```python
from build123d import *

# Parameters (mm, degrees)
SKETCH1_W           = 307
SKETCH1_H           = 115
BOSS_EXTRUDE1_DEPTH = 4
CUT_EXTRUDE1_DEPTH  = 4
SKETCH3_W           = 4
SKETCH3_H           = 40.5
SKETCH3_H_2         = 38.5
CUT_EXTRUDE2_DEPTH  = 4
SKETCH4_W           = 46.333333333
SKETCH4_H           = 4
SKETCH4_W_2         = 42.33
BOSS_EXTRUDE3_DEPTH = 4
SKETCH5_W           = 36
SKETCH5_H           = 4
BOSS_EXTRUDE4_DEPTH = 4
SKETCH7_W           = 22.24
SKETCH7_H           = 4
BOSS_EXTRUDE6_DEPTH = 4
SKETCH8_W           = 4
SKETCH8_H           = 38
CUT_EXTRUDE3_DEPTH  = 4
LPATTERN1_COUNT     = 3
LPATTERN1_PITCH     = 72
SKETCH9_W           = 70
SKETCH9_H           = 4
BOSS_EXTRUDE7_DEPTH = 4
CUT_EXTRUDE4_DEPTH  = 4
LPATTERN2_COUNT     = 2
LPATTERN2_PITCH     = 84
LPATTERN3_COUNT     = 2
LPATTERN3_PITCH     = 194
SKETCH11_W          = 4
SKETCH11_H          = 3.457617008
BOSS_EXTRUDE8_DEPTH = 4


with BuildPart() as part:
    # Sketch1 → Boss-Extrude1 (new body)
    with BuildSketch(Plane(origin=(0, 0, 0), x_dir=(0, 0, -1), z_dir=(1, 0, 0))):
        with Locations((153.5, 57.5)):
            Rectangle(SKETCH1_W, SKETCH1_H)
    extrude(amount=BOSS_EXTRUDE1_DEPTH)

    # Sketch2 → Cut-Extrude1 (cut)
    with BuildSketch(Plane.ZY):
        with BuildLine():
            Line((-78.216729868, 30.591924331), (-78.216729868, 118.288831206))
            Line((-78.216729868, 118.288831206), (-68.216729868, 118.288831206))
            Line((-68.216729868, 118.288831206), (-68.216729868, 30.591924331))
            ThreePointArc((-68.216729868, 30.591924331), (-73.216729868, 25.591924331), (-78.216729868, 30.591924331))
        make_face()
    extrude(amount=-CUT_EXTRUDE1_DEPTH, mode=Mode.SUBTRACT)

    # Sketch3 → Cut-Extrude2 (cut)
    with BuildSketch(Plane.ZY):
        with Locations((-2, 16.25)):
            Rectangle(SKETCH3_W, SKETCH3_H)
        with Locations((-2, 95.75)):
            Rectangle(SKETCH3_W, SKETCH3_H_2)
    extrude(amount=-CUT_EXTRUDE2_DEPTH, mode=Mode.SUBTRACT)

    # Sketch4 → Boss-Extrude3 (add)
    with BuildSketch(Plane.ZY):
        with Locations((-283.833333334, -2)):
            Rectangle(SKETCH4_W, SKETCH4_H)
        with Locations((-25.165, -2)):
            Rectangle(SKETCH4_W_2, SKETCH4_H)
    extrude(amount=-BOSS_EXTRUDE3_DEPTH)

    # Sketch5 → Boss-Extrude4 (add)
    with BuildSketch(Plane.ZY):
        with Locations((-271, 117)):
            Rectangle(SKETCH5_W, SKETCH5_H)
    boss_extrude4 = extrude(amount=-BOSS_EXTRUDE4_DEPTH)

    # Sketch7 → Boss-Extrude6 (add)
    with BuildSketch(Plane.ZY):
        with Locations((-34.856729868, 117)):
            Rectangle(SKETCH7_W, SKETCH7_H)
    extrude(amount=-BOSS_EXTRUDE6_DEPTH)

    # Sketch8 → Cut-Extrude3 (cut)
    with BuildSketch(Plane.ZY):
        with Locations((-305, 56.5)):
            Rectangle(SKETCH8_W, SKETCH8_H)
    extrude(amount=-CUT_EXTRUDE3_DEPTH, mode=Mode.SUBTRACT)

    # LPattern1: Boss-Extrude4 ×3
    with Locations(*[(0, 0, i * LPATTERN1_PITCH) for i in range(1, LPATTERN1_COUNT)]):
        add(boss_extrude4)

    # Sketch9 → Boss-Extrude7 (add)
    with BuildSketch(Plane.ZY):
        with Locations((-153.666666667, -2)):
            Rectangle(SKETCH9_W, SKETCH9_H)
    extrude(amount=-BOSS_EXTRUDE7_DEPTH)

    # Sketch10 → Cut-Extrude4 (cut)
    with BuildSketch(Plane.ZY):
        with BuildLine():
            Line((-245, 97.5), (-245, 17.5))
            ThreePointArc((-245, 17.5), (-247, 15.5), (-249, 17.5))
            Line((-249, 17.5), (-249, 97.5))
            ThreePointArc((-249, 97.5), (-247, 99.5), (-245, 97.5))
        make_face()
        with BuildLine():
            Line((-240.5, 97.5), (-240.5, 17.5))
            ThreePointArc((-240.5, 17.5), (-238.5, 15.5), (-236.5, 17.5))
            Line((-236.5, 17.5), (-236.5, 97.5))
            ThreePointArc((-236.5, 97.5), (-238.5, 99.5), (-240.5, 97.5))
        make_face()
        with BuildLine():
            Line((-232, 97.5), (-232, 17.5))
            ThreePointArc((-232, 17.5), (-230, 15.5), (-228, 17.5))
            Line((-228, 17.5), (-228, 97.5))
            ThreePointArc((-228, 97.5), (-230, 99.5), (-232, 97.5))
        make_face()
    cut_extrude4 = extrude(amount=-CUT_EXTRUDE4_DEPTH, mode=Mode.SUBTRACT)

    # LPattern2: Cut-Extrude4 ×2
    with Locations(*[(0, 0, i * LPATTERN2_PITCH) for i in range(1, LPATTERN2_COUNT)]):
        add(cut_extrude4, mode=Mode.SUBTRACT)

    # LPattern3: Cut-Extrude4 ×2
    with Locations(*[(0, 0, i * LPATTERN3_PITCH) for i in range(1, LPATTERN3_COUNT)]):
        add(cut_extrude4, mode=Mode.SUBTRACT)

    # Sketch11 → Boss-Extrude8 (add)
    with BuildSketch(Plane(origin=(0, 115, 0), x_dir=(1, 0, 0), z_dir=(0, 1, 0))):
        with Locations((2, 305.271191496)):
            Rectangle(SKETCH11_W, SKETCH11_H)
    extrude(amount=BOSS_EXTRUDE8_DEPTH)


solid = part.part
```
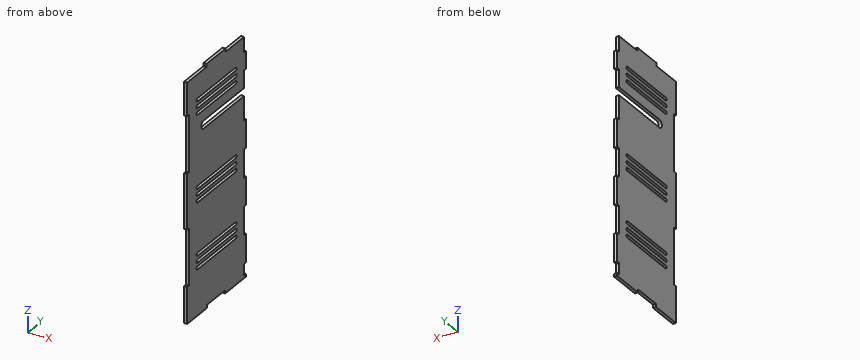
CAD build for the part. Positions are in the model's coordinates, mm. Round coordinates to 2 decimals unless told otherwise and drop trailing zeros. Order: outer loops, then holes, each group sorted by start corner. A loop starts at its lowest first (then second) coordinate and runs counter-clockwise, first axis right, second up. Notation, with made-up numbers: (43, 38.5) - (48, 38.5) arc R37 cw to (48, 76.5) - close; hole circle Ø8 at (34.25, 64.5). An arc over 180 degrees is marked (long way). Answer as CSV lines item,"result". Start each with the question number.
1. Saw through at A-A, the plane y = 109. Write the cut outline in (x, z), and give its area (3 significant figures).
2. Saw through at B-B, the plane x = 2.6. Count the separate pieces of the cut face and the enclosed holes in it, and give its area (3 significant figures).
3. Drill centre lines: L1, parallel to Z at x = 3.15, y = 113.5; L2, parallel to Y at x = 1.4, z = -250; L3, parallel to Y at x = 1.75, z = -169. Where is each one in solid material? Low to high. Write a range as [from, to].
4. Pin check, flat tips, straight feed: pin 1 (1.2 mm diameter, centred on x = 2.5, y = 58, fed in from -Z); pin 2 (2 mm diameter, centred on x = 2.5, y = 7, fed in from +Z); pin 3 (2 mm diameter, centred on x = 2, z = -230, fed in from +Y). Stop position of each tip, or through.
Model answer:
1,outline,"(0, -307) - (4, -307) - (4, -78.22) - (0, -78.22) - close; (0, -68.22) - (4, -68.22) - (4, -4) - (0, -4) - close"
1,area,"1,170 mm²"
2,separate pieces,"1"
2,enclosed holes,"9"
2,area,"32,100 mm²"
3,L1,"z = [-307, -78.22], [-68.22, -4]"
3,L2,"y = [0, 115]"
3,L3,"y = [-4, 115]"
4,pin 1,"stops at z = -303"
4,pin 2,"stops at z = -4"
4,pin 3,"stops at y = 115"
